Read the model definition and answer for the solid it produces. Units are mm, in the model's axes. A direction names the side the tool comes from. Coordinates: 2 decimals unless noted, no trailing zeros. Write each loop counter-clockwise with the first axis right and the second up, starting at its lowest first coordinate (ties: lowest second). Pieces come first, ordered by that corner, then holes.
Item 1: Section B-B (x = -8) is taken. Give the vertices of the cut face in (y, z).
Item 2: Determine the mould class of faces 6 (the face through (-32, 0, -45)), 7 (the face through (-21.348, 37.675, -2.958)), 8 (the face through (-1, 1, -6)) for opening direction X: released by +X, released by -X, zero draft, split by the parting line, or undercut.
Item 3: Section C-C (y = 23.5) is taken. Give the vertices of the cut face in (x, z).
Item 4: A tool of negligible diameter and unlimited length cuts with its end or side. For faces 1 (the face through (33, -17.5, -25)), 2 (the face through (33, 17.5, -25)), 3 (the face through (-30.7, 0, -27)), 4 (the face through (-34.2, 0, -26)), 5 (the face through (34.2, 0, -25)), from which of +Z, -Z, +X, -X, +Y, -Y can it reach the whole face along a straight path? Write none if from no direction.
Item 5: Straight lines are drawn through the part: probe 1 along Y at (x, z) = (32.15, -27); probe 2 along X at (y, z) = (5, -39); probe 3 along Y at (x, z) = (32.5, -39.5). For each, find the intervals that lie inside material, in ascending order.
Item 6: Each of these flat-tipped pins is pushed along its axis until it touches: P1, Ø1.7, axis at y = 0, z = -39.5, coming from the +X side; P2, Ø2.5, axis at y = 12.5, z = -27, coming from the -X side; P3, Ø6, axis at x = 31.5, z = -27.5, coming from the +Y side. Where does it stop, or does it pass through?
Item 7: Section A-A (y = -2) is taken. Give the vertices of the cut face in (x, z).
from build123d import *

# Parameters (mm, degrees)
BOSS_EXTRUDE1_DEPTH = 17.5
SKETCH2_R           = 0.75
CUT_EXTRUDE1_DEPTH  = 68.4
SKETCH2_3_R         = 0.75
CUT_EXTRUDE2_DEPTH  = 69.4
SKETCH3_W           = 82.6
SKETCH3_H           = 35
BOSS_EXTRUDE2_DEPTH = 6
BOSS_EXTRUDE3_DEPTH = 6


with BuildPart() as part:
    # Sketch1 → Boss-Extrude1 (new body, symmetric)
    with BuildSketch(Plane(origin=(0, 0, 0), x_dir=(1, 0, 0), z_dir=(0, 1, 0))):
        with BuildLine():
            Line((-29.2, 0), (29.2, 0))
            ThreePointArc((29.2, 0), (32.735533906, 1.464466094), (34.2, 5))
            Line((34.2, 5), (34.2, 45))
            Line((34.2, 45), (30.7, 45))
            Line((30.7, 45), (30.7, 10))
            ThreePointArc((30.7, 10), (29.235533906, 6.464466094), (25.7, 5))
            Line((25.7, 5), (-25.7, 5))
            ThreePointArc((-25.7, 5), (-29.235533906, 6.464466094), (-30.7, 10))
            Line((-30.7, 10), (-30.7, 45))
            Line((-30.7, 45), (-34.2, 45))
            Line((-34.2, 45), (-34.2, 5))
            ThreePointArc((-34.2, 5), (-32.735533906, 1.464466094), (-29.2, 0))
        make_face()
    extrude(amount=BOSS_EXTRUDE1_DEPTH, both=True)

    # Sketch2 → Cut-Extrude1 (cut)
    with BuildSketch(Plane.ZY.offset(34.2)):
        with Locations((-27, 12.5)):
            Circle(SKETCH2_R)
        with Locations((-18.161165235, 8.838834765)):
            Circle(SKETCH2_R)
        with Locations((-14.5, 0)):
            Circle(SKETCH2_R)
        with Locations((-18.161165235, -8.838834765)):
            Circle(SKETCH2_R)
        with Locations((-35.838834765, -8.838834765)):
            Circle(SKETCH2_R)
        with Locations((-39.5, 0)):
            Circle(SKETCH2_R)
        with Locations((-35.838834765, 8.838834765)):
            Circle(SKETCH2_R)
    extrude(amount=-CUT_EXTRUDE1_DEPTH, mode=Mode.SUBTRACT)

    # Sketch2<3> → Cut-Extrude2 (cut, through all)
    with BuildSketch(Plane.ZY.offset(34.2)):
        with Locations((-27, -12.5)):
            Circle(SKETCH2_3_R)
    extrude(amount=-CUT_EXTRUDE2_DEPTH, mode=Mode.SUBTRACT)

    # Sketch3 → Boss-Extrude2 (add)
    with BuildSketch(Plane.XY):
        Rectangle(SKETCH3_W, SKETCH3_H)
    extrude(amount=-BOSS_EXTRUDE2_DEPTH)

    # Sketch5 → Boss-Extrude3 (add)
    with BuildSketch(Plane.XY):
        Polygon((43.301270189, 25), (0, 50), (-43.301270189, 25), (-43.301270189, -25), (0, -50), (43.301270189, -25), align=None)
    extrude(amount=-BOSS_EXTRUDE3_DEPTH)


solid = part.part
Established:
1. outline: (-45.38, -6) - (45.38, -6) - (45.38, 0) - (-45.38, 0) - close
2. face 6: zero draft
2. face 7: released by -X
2. face 8: undercut
3. outline: (-43.3, -6) - (43.3, -6) - (43.3, 0) - (-43.3, 0) - close
4. face 1: -Z, +X, -X, -Y
4. face 2: -Z, +X, -X, +Y
4. face 3: -Z, +Y, -Y
4. face 4: -Z, -X, +Y, -Y
4. face 5: -Z, +X, +Y, -Y
5. probe 1: y = -17.5 to -13.25, -11.75 to 11.75, 13.25 to 17.5
5. probe 2: x = -34.2 to -30.7, 30.7 to 34.2
5. probe 3: y = -17.5 to -0.75, 0.75 to 17.5
6. P1: stops at x = 34.2
6. P2: stops at x = -34.2
6. P3: stops at y = 17.5
7. outline: (-43.3, -6) - (-34.2, -6) - (-34.2, -45) - (-30.7, -45) - (-30.7, -10) arc R5 cw to (-28.7, -6) - (28.7, -6) arc R5 cw to (30.7, -10) - (30.7, -45) - (34.2, -45) - (34.2, -6) - (43.3, -6) - (43.3, 0) - (-43.3, 0) - close
